Design review of the part built by this model. Coordinates are the model's own, in mm. Face numbers are marked on the shaded views. A direction names the side the tool comes from. Give positions to 0.01 mm unless a question says otherwise; leave off trailing zeros. Write each loop counter-clockwise with the first axis right and the second up, starting at its lowest first coordinate (ties: lowest second). Pieces come first, ordered by that corner, then holes.
```python
from build123d import *

# Parameters (mm, degrees)
F0_W      = 76.2
F0_H      = 101.6
F1_DEPTH  = 15.0114
F2_R      = 2.54
F3_DEPTH  = 101.601
F4_R      = 5.08
F5_DEPTH  = 88.9
F7_DEPTH  = 6.2484
F8_R      = 2.54
F9_DEPTH  = 69.9526
F10_R     = 5.08
F11_DEPTH = 63.5


with BuildPart() as f1:
    # F0 (on Top) → F1 (new body)
    with BuildSketch(Plane.XY):
        Rectangle(F0_W, F0_H)
    extrude(amount=F1_DEPTH)

    # F2 (on face) → F3 (cut, through all)
    with BuildSketch(Plane.XZ.offset(50.8)):
        with Locations((-12.7, 8.6614)):
            Circle(F2_R)
        with Locations((12.7, 8.6614)):
            Circle(F2_R)
    extrude(amount=-F3_DEPTH, mode=Mode.SUBTRACT)

    # F4 (on face) → F5 (cut, through all)
    with BuildSketch(Plane.XZ.offset(50.8)):
        with Locations((-12.7, 8.6614)):
            Circle(F4_R)
        with Locations((12.7, 8.6614)):
            Circle(F4_R)
    extrude(amount=-F5_DEPTH, mode=Mode.SUBTRACT)

    # F6 (on face) → F7 (cut)
    with BuildSketch(Plane.YZ.offset(38.1)):
        Polygon((-15.0749, 11.1238474629), (-17.4498, 7.0104), (-15.0749, 2.8969525371), (-10.3251, 2.8969525371), (-7.9502, 7.0104), (-10.3251, 11.1238474629), align=None)
        Polygon((10.3251, 11.1238474629), (7.9502, 7.0104), (10.3251, 2.8969525371), (15.0749, 2.8969525371), (17.4498, 7.0104), (15.0749, 11.1238474629), align=None)
    extrude(amount=-F7_DEPTH, mode=Mode.SUBTRACT)

    # F8 (on face) → F9 (cut, through all)
    with BuildSketch(Plane.YZ.offset(31.8516)):
        with Locations((-12.7, 7.0104)):
            Circle(F8_R)
        with Locations((12.7, 7.0104)):
            Circle(F8_R)
    extrude(amount=-F9_DEPTH, mode=Mode.SUBTRACT)

    # F10 (on face) → F11 (cut, through all)
    with BuildSketch(Plane(origin=(-38.1, 0, 0), x_dir=(0, -1, 0), z_dir=(-1, 0, 0))):
        with Locations((-12.7, 7.0104)):
            Circle(F10_R)
        with Locations((12.7, 7.0104)):
            Circle(F10_R)
    extrude(amount=-F11_DEPTH, mode=Mode.SUBTRACT)


solid = f1.part
```
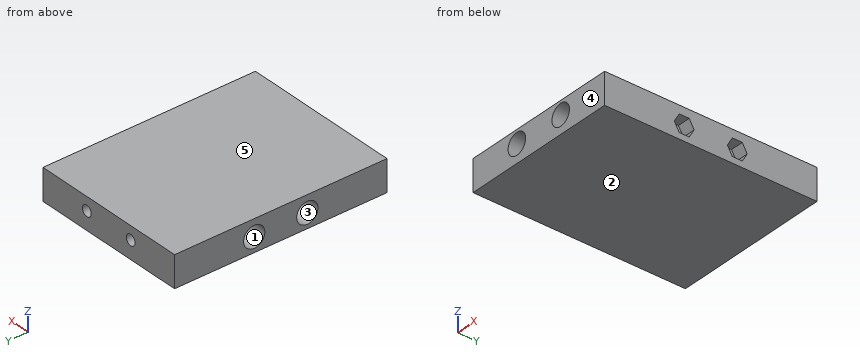
(1) Mouldability with a two-part tool opening along Z and no side actions: class the marked faces 3, 4 and 5 as pulls with the +Z half, pulls with the -Z half, needs draft (parallel to the pull), parting line crosses it, or undercut.
Resolved:
face 3: undercut
face 4: needs draft
face 5: pulls with the +Z half
(2) Clearance check with flat-ended pins moving along their axes: P1, Ø6, axis at y = 12.7, z = 7.01, coming from the -X side; P2, Ø5, axis at x = 36, y = -13.5, coming from the -Z side; P3, Ø8, axis at x = -12.7, z = 8.66, coming from the -Y side. State where each tip first meets the part, or that it passes through.
Resolved:
P1: stops at x = 25.4
P2: stops at z = 0
P3: stops at y = 38.1
(3) Consider section A-A, the plane x = 12.7. Give the boundary of the cut face in (y, z), then the cut area to 3 significant figures.
Resolved:
outline: (-50.8, 0) - (50.8, 0) - (50.8, 6.12) - (38.1, 6.12) - (38.1, 3.58) - (16.45, 3.58) arc R5.08 cw to (8.95, 3.58) - (-8.95, 3.58) arc R5.08 cw to (-16.45, 3.58) - (-50.8, 3.58) - close; (-50.8, 13.74) - (38.1, 13.74) - (38.1, 11.2) - (50.8, 11.2) - (50.8, 15.01) - (-50.8, 15.01) - close
area: 540 mm2
(4) Consider section C-C, the plane y = -12.7. Give the boundary of the cut face in (x, z), then the cut area to 3 significant figures.
Resolved:
outline: (-38.1, 0) - (38.1, 0) - (38.1, 2.9) - (31.85, 2.9) - (31.85, 4.47) - (25.4, 4.47) - (25.4, 1.93) - (-38.1, 1.93) - close; (-38.1, 12.09) - (-16.45, 12.09) arc R5.08 cw to (-8.95, 12.09) - (8.95, 12.09) arc R5.08 cw to (16.45, 12.09) - (25.4, 12.09) - (25.4, 9.55) - (31.85, 9.55) - (31.85, 11.12) - (38.1, 11.12) - (38.1, 15.01) - (-38.1, 15.01) - close
area: 397 mm2
(5) To check wall thickness, follow L1, parallel to X at y = 30, z = 10.5; L2, parallel to X at y = -29, z = 4.5; L3, parallel to Y at x = -21, z = 10.75. State the ranges of each line that lie inside material, in increasing order.
Resolved:
L1: x = -38.1 to -17.44, -7.96 to 7.96, 17.44 to 38.1
L2: x = -38.1 to -15.61, -9.79 to 9.79, 15.61 to 38.1
L3: y = -50.8 to -16.14, -9.26 to 9.26, 16.14 to 50.8
(6) Consider section D-D, the plane y = 34.5. Give the boundary of the cut face in (x, z), then the cut area to 3 significant figures.
Resolved:
outline: (-38.1, 0) - (38.1, 0) - (38.1, 15.01) - (-38.1, 15.01) - close; hole circle Ø10.16 at (-12.7, 8.66); hole circle Ø10.16 at (12.7, 8.66)
area: 982 mm2
(7) Tool access review of the marked faces 1 and 2: name each direction out of +Z, -Z, +X, -X, +Y, -Y from which nothing blocks a thin tool from reaching the whole face with its end or side.
Resolved:
face 1: -X
face 2: -Z, +X, -X, +Y, -Y
(8) Consider section B-B, the plane x = 3. Give the boundary of the cut face in (y, z), then the cut area to 3 significant figures.
Resolved:
outline: (-50.8, 0) - (50.8, 0) - (50.8, 15.01) - (-50.8, 15.01) - close; hole circle Ø10.16 at (-12.7, 7.01); hole circle Ø10.16 at (12.7, 7.01)
area: 1,360 mm2
